Check sheet for the modelled part. Datum: model origin and axes. Units: mm. A direction names the side the tool comes from. Round coordinates to 2 decimals unless told otherwise and drop trailing zeros. Write each loop counter-clockwise with the first axis right and the second up, starting at its lowest first coordinate (ties: lowest second). Pieces come first, ordered by that corner, then holes. Notation, with made-up numbers: (60.25, 46) -> (85.25, 46) arc R28 ccw to (85.25, 83) -> close; hole circle Ø10 at (26, 46). An arc over 180 degrees is marked (long way). One line per item, written item: value.
from build123d import *

# Parameters (mm, degrees)
F0_W     = 9.525
F0_H     = 77.75448
F1_DEPTH = 15.875
F2_W     = 12.4875006322
F2_H     = 50
F3_DEPTH = 25
F5_DEPTH = 1
F7_DEPTH = 1
F9_DEPTH = 1


with BuildPart() as f1:
    # F0 (on Front) → F1 (new body)
    with BuildSketch(Plane.XZ):
        Rectangle(F0_W, F0_H)
    extrude(amount=F1_DEPTH)

    # F2 (on face) → F3 (cut)
    with BuildSketch(Plane.YZ.offset(4.7625)):
        with Locations((-9.6312496839, -13.87724)):
            Rectangle(F2_W, F2_H)
    extrude(amount=-F3_DEPTH, mode=Mode.SUBTRACT)

    # F4 (on face) → F5 (join)
    with BuildSketch(Plane(origin=(-4.7625, 0, 0), x_dir=(0, -1, 0), z_dir=(-1, 0, 0))):
        Polygon((0, 11.12276), (3.3874993678, 11.12276), (15.875, 11.12276), (15.875, 38.87724), (0, 38.87724), align=None)
    extrude(amount=F5_DEPTH)

    # F6 (on face) → F7 (join)
    with BuildSketch(Plane.YZ.offset(4.7625)):
        Polygon((-15.875, 11.12276), (-3.3874993678, 11.12276), (0, 11.12276), (0, 38.87724), (-15.875, 38.87724), align=None)
    extrude(amount=F7_DEPTH)

    # F8 (on face) → F9 (join)
    with BuildSketch(Plane(origin=(0, 0, 0), x_dir=(-1, 0, 0), z_dir=(0, 1, 0))):
        Polygon((-5.7625, 38.87724), (-5.7625, 11.12276), (-4.7625, 11.12276), (4.7625, 11.12276), (5.7625, 11.12276), (5.7625, 38.87724), align=None)
    extrude(amount=F9_DEPTH)


solid = f1.part
Item 1: Sectioned sample at A-A (y = -1.25). Enter the section's corners in (x, z).
Result set:
outline: (-5.76, 11.12) -> (-4.76, 11.12) -> (-4.76, -38.88) -> (4.76, -38.88) -> (4.76, 11.12) -> (5.76, 11.12) -> (5.76, 38.88) -> (-5.76, 38.88) -> close
Item 2: Sectioned sample at B-B (x = -1.5). Enter the section's corners in (y, z) (1 decimal).
Result set:
outline: (-15.9, 11.1) -> (-3.4, 11.1) -> (-3.4, -38.9) -> (0, -38.9) -> (0, 11.1) -> (1, 11.1) -> (1, 38.9) -> (-15.9, 38.9) -> close
Item 3: Depth check by flat-ended pin: pin 1 (1.7 mm diameter, centred on y = -1.5, z = -4.5, fed in from +X); pin 2 (3 mm diameter, centred on x = 0, y = -9, fed in from -Z); pin 3 (1.5 mm diameter, centred on x = -1.5, z = -14.5, fed in from +Y). Enter the tip coordinate at first touch or a pass-through.
Result set:
pin 1: x = 4.76
pin 2: z = 11.12
pin 3: y = 0
Item 4: Sectioned sample at D-D (y = -6.75). Enter the section's corners in (x, z).
Result set:
outline: (-5.76, 11.12) -> (5.76, 11.12) -> (5.76, 38.88) -> (-5.76, 38.88) -> close
Item 5: Sectioned sample at C-C (z = -18.5). Enter the section's corners in (x, y), then the cut area to 3 significant figures.
Result set:
outline: (-4.76, -3.39) -> (4.76, -3.39) -> (4.76, 0) -> (-4.76, 0) -> close
area: 32.3 mm^2
Item 6: Material ranges on line 1 along Y through (x, z) = (-0.25, 7); line 2 along Z through (x, y) = (5, -8.5), recorded low to high.
Result set:
line 1: -3.39 to 0
line 2: 11.12 to 38.88
Item 7: Tool access check on faces 1 (the flat face through (0, -3.387, -14)), 2 (the flat face through (0, 0, -14)), 3 (the flat face through (0, -15.875, 25)), 4 (the flat face through (-4.762, -2, -14)), 5 (the flat face through (4.762, -2, -14)). Record the directions out of +Z, -Z, +X, -X, +Y, -Y that give a thin tool (end or side, any length) a straight path to the whole face; none if there is none.
Result set:
face 1: -Z, +X, -X, -Y
face 2: -Z, +X, -X, +Y
face 3: +Z, -Z, +X, -X, -Y
face 4: -Z, -X, +Y, -Y
face 5: -Z, +X, +Y, -Y
